Here's how the part is built. I have some questions about the finished solid (model axes, mm). A direction names the side the tool comes from. Coordinates: 2 decimals unless noted, no trailing zeros. Write each loop counter-clockwise with the first axis right and the second up, starting at its lowest first coordinate (ties: lowest second). Pieces come first, ordered by that corner, then holes. Notation, with made-up numbers: (-12, 79) -> (31, 79) arc R31 ccw to (31, 106) -> close; hole circle Ø8 at (40.5, 16). An arc over 180 degrees is marked (long way). Use a Markdown table: item, result. Add a question column.
Item 1: On a 3-axis mill with a long thin cutter (end or side, diameter ignored), from which of +Z, -Z, +X, -X, +Y, -Y can I reach the whole of each face in a straight line? I mean faces 4 (the cylindrical face through (51.574, 2.465, 9.19)), 5 (the flat face through (65, 9, 14)), 6 (the flat face through (64, 2, 20)), 7 (the cylindrical face through (44.08, 14.7, 3.45)). Say none if no direction works.
Item 2: Will these pins go through, and if not, where does the flat tip stop? pin 1 Ø5 at (x, y) = (31.5, 9.5) entering from +Z; pin 2 Ø3 at (x, z) = (53.5, 9) entering from +Y; pin 3 Ø4 at (x, z) = (63, 4.5) entering from -Y.
Item 3: If we mould it in two halves opening along X, with no side actions, what happens to faces 1 (the flat face through (9, 30, 3)), 2 (the cylindrical face through (12.355, 2.465, 11.133)), 3 (the flat face through (70, 11, 8))? For each: pulls with the +X half, pulls with the -X half, needs draft (parallel to the pull), parting line crosses it, or undercut.
Item 4: Imagine slicing it at C-C, the plane y = 9.75. Write out the boundary of the cut face in (x, z).
Item 5: Imagine slicing it at A-A, the plane z = 5.25. Write out the boundary of the cut face in (x, y), and give its area (3 significant figures).
Item 6: If I drill on line 1 along X through (y, z) = (14.75, 13.25); line 2 along X through (y, z) = (3.75, 11.25); line 3 along X through (y, z) = (12.5, 3.5), over which ranges is the centre line in solid material (lowest first)? Write a range as from..to.
Item 7: Imagine slicing it at D-D, the plane x = 31.2. Write out the boundary of the cut face in (y, z), and give its area (3 significant figures).
Item 8: Imagine slicing it at B-B, the plane y = 3.5. Write out the boundary of the cut face in (x, z).
```python
from build123d import *

# Parameters (mm, degrees)
SKETCH1_W           = 70
SKETCH1_H           = 30
BOSS_EXTRUDE1_DEPTH = 20
CUT_EXTRUDE2_DEPTH  = 21
CUT_EXTRUDE3_DEPTH  = 71
CUT_EXTRUDE7_DEPTH  = 31
BOSS_EXTRUDE3_DEPTH = 5
CUT_EXTRUDE8_DEPTH  = 71


with BuildPart() as part:
    # Sketch1 → Boss-Extrude1 (new body)
    with BuildSketch(Plane.XY):
        with Locations((-35, 15)):
            Rectangle(SKETCH1_W, SKETCH1_H)
    boss_extrude1 = extrude(amount=BOSS_EXTRUDE1_DEPTH)

    # Sketch1_3 → Cut-Extrude2 (cut, through all)
    with BuildSketch(Plane.XY):
        with BuildLine():
            Line((-18.200000763, 30), (-44.200000763, 30))
            ThreePointArc((-44.200000763, 30), (-31.200000763, 15), (-18.200000763, 30))
        make_face()
        with BuildLine():
            ThreePointArc((-15.706172943, 15.55638361), (-14.370568008, 14.668173822), (-13.850757599, 13.150756836))
            ThreePointArc((-13.850757599, 13.150756836), (-18.325338895, 11.617932335), (-15.706172943, 15.55638361))
        make_face()
        with BuildLine():
            ThreePointArc((-45.615119934, 15.61277771), (-44.064114621, 14.676308172), (-43.56823349, 12.933696747))
            ThreePointArc((-43.56823349, 12.933696747), (-48.042503261, 11.636717399), (-45.615119934, 15.61277771))
        make_face()
    cut_extrude2 = extrude(amount=CUT_EXTRUDE2_DEPTH, mode=Mode.SUBTRACT)

    # Sketch2 → Cut-Extrude3 (cut, through all)
    with BuildSketch(Plane.ZY.offset(70)):
        Polygon((20, 30), (7, 30), (20, 5), align=None)
    cut_extrude3 = extrude(amount=-CUT_EXTRUDE3_DEPTH, mode=Mode.SUBTRACT)

    # Mirror1: Boss-Extrude1, Cut-Extrude2, Cut-Extrude3 across plane
    add(boss_extrude1.mirror(Plane(origin=(0, 30, 20), x_dir=(0, 0, 1), z_dir=(1, 0, 0))))
    add(cut_extrude2.mirror(Plane(origin=(0, 30, 20), x_dir=(0, 0, 1), z_dir=(1, 0, 0))), mode=Mode.SUBTRACT)
    add(cut_extrude3.mirror(Plane(origin=(0, 30, 20), x_dir=(0, 0, 1), z_dir=(1, 0, 0))), mode=Mode.SUBTRACT)

    # Sketch4 → Cut-Extrude7 (cut, through all)
    with BuildSketch(Plane(origin=(0, 0, 0), x_dir=(1, 0, 0), z_dir=(0, 1, 0))):
        with BuildLine():
            Line((5, -11.999999865), (5, -20))
            Line((5, -20), (65, -20))
            Line((65, -20), (65, -12))
            ThreePointArc((65, -12), (63.535533906, -8.464466094), (60, -7))
            Line((60, -7), (22.686811447, -7))
            Line((22.686811447, -7), (21.717826843, -7.061558247))
            Line((21.717826843, -7.061558247), (10, -7))
            ThreePointArc((10, -7), (6.464466102, -8.464466007), (5, -11.999999865))
        make_face()
    extrude(amount=CUT_EXTRUDE7_DEPTH, mode=Mode.SUBTRACT)

    # Sketch4_6 → Boss-Extrude3 (add)
    with BuildSketch(Plane(origin=(0, 0, 0), x_dir=(1, 0, 0), z_dir=(0, 1, 0))):
        with BuildLine():
            Line((57.5, -20), (65, -20))
            Line((65, -20), (65, -12))
            ThreePointArc((65, -12), (63.535533906, -8.464466094), (60, -7))
            Line((60, -7), (47.881000272, -7))
            ThreePointArc((47.881000272, -7), (51.610779808, -9.240727474), (52.5, -13.5))
            ThreePointArc((52.5, -13.5), (53.428531793, -17.958821698), (57.5, -20))
        make_face()
        with BuildLine():
            ThreePointArc((58.071636237, -15.298134071), (57.54254335, -11.279271131), (61.499999792, -10.401924497))
            ThreePointArc((61.499999792, -10.401924497), (62.999999734, -13.000000826), (61.499999759, -15.598077136))
            ThreePointArc((61.499999759, -15.598077136), (59.738532149, -15.988585106), (58.071636237, -15.298134071))
        make_face(mode=Mode.SUBTRACT)
        with BuildLine():
            Line((5, -11.999999865), (5, -20))
            Line((5, -20), (12.5, -20))
            ThreePointArc((12.5, -20), (16.552378538, -17.944137337), (17.5, -13.5))
            ThreePointArc((17.5, -13.5), (18.286173232, -9.293081984), (21.929830501, -7.048089949))
            Line((21.929830501, -7.048089949), (21.717826843, -7.061558247))
            Line((21.717826843, -7.061558247), (10, -7))
            ThreePointArc((10, -7), (6.464466102, -8.464466007), (5, -11.999999865))
        make_face()
        with BuildLine():
            ThreePointArc((7.045577049, -13.520944595), (7.401923496, -11.500000278), (8.973938942, -10.180922508))
            ThreePointArc((8.973938942, -10.180922508), (12.387007699, -11.175196953), (12.37415177, -14.730116746))
            ThreePointArc((12.37415177, -14.730116746), (9.302656578, -15.920012423), (7.045577049, -13.520944595))
        make_face(mode=Mode.SUBTRACT)
    extrude(amount=BOSS_EXTRUDE3_DEPTH)

    # Sketch11 → Cut-Extrude8 (cut, through all)
    with BuildSketch(Plane(origin=(0, 0, 0), x_dir=(0, 0, -1), z_dir=(1, 0, 0))):
        Polygon((-20, 0), (0, 0), (0, 30), (-7, 30), (-20, 5), align=None)
    extrude(amount=-CUT_EXTRUDE8_DEPTH, mode=Mode.SUBTRACT)


solid = part.part
```
Ans:
| question | item | result |
|---|---|---|
| 1 | face 4 | +Y, -Y |
| 1 | face 5 | +Z, +Y |
| 1 | face 6 | +Z, +X, -X, +Y, -Y |
| 1 | face 7 | +Z, -Z |
| 2 | pin 1 | stops at z = 7 |
| 2 | pin 2 | stops at y = 5 |
| 2 | pin 3 | stops at y = 0 |
| 3 | face 1 | needs draft |
| 3 | face 2 | undercut |
| 3 | face 3 | pulls with the +X half |
| 4 | outline | (0, 0) -> (70, 0) -> (70, 17.53) -> (65, 17.53) -> (65, 12) arc R5 cw to (60, 7) -> (22.69, 7) -> (21.72, 7.06) -> (10, 7) arc R5 cw to (5, 12) -> (5, 17.53) -> (0, 17.53) -> close |
| 5 | outline | (0, 0) -> (70, 0) -> (70, 30) -> (44.2, 30) arc R13.13 cw (long way) to (18.2, 30) -> (0, 30) -> close; hole circle Ø4.99 at (16.35, 13.14); hole (43.57, 12.93) arc R2.5 ccw (long way) to (45.62, 15.61) arc R2.47 ccw to start |
| 5 | area | 1,740 mm^2 |
| 6 | line 1 | x = 0..5, 65..70 |
| 6 | line 2 | x = 0..7.56, 12.44..17.46, 52.49..57.56, 62.44..70 |
| 6 | line 3 | x = 0..13.93, 18.76..43.65, 48.47..70 |
| 7 | outline | (0, 0) -> (15, 0) -> (15, 7) -> (0, 7) -> close |
| 7 | area | 105 mm^2 |
| 8 | outline | (0, 0) -> (70, 0) -> (70, 20) -> (57.5, 20) arc R5.23 ccw to (52.5, 13.5) arc R5.43 cw to (47.88, 7) -> (22.69, 7) -> (21.93, 7.05) arc R5.28 cw to (17.5, 13.5) arc R5.27 ccw to (12.5, 20) -> (0, 20) -> close; hole (7.05, 13.52) arc R3 ccw to (8.97, 10.18) arc R2.95 ccw to (12.37, 14.73) arc R2.95 ccw to start; hole circle Ø6 at (60, 13) |
